from build123d import *

# Parameters (mm, degrees)
RESSALTO_EXTRUS_O1_DEPTH = 5


with BuildPart() as part:
    # Esboço1 → Ressalto-extrusão1 (new body)
    with BuildSketch(Plane.XY):
        with BuildLine():
            Line((0, 26.5), (0, 55.5))
            ThreePointArc((0, 55.5), (-9.054313021, 54.756455471), (-17.86602118, 52.545744711))
            Line((-17.86602118, 52.545744711), (-27.213841848, 24.565961853))
            Line((-27.213841848, 24.565961853), (-25.202997682, 8.188950351))
            Line((-25.202997682, 8.188950351), (-52.783636654, 17.150443188))
            ThreePointArc((-52.783636654, 17.150443188), (-54.874420381, 8.309511893), (-55.494877077, -0.754067766))
            Line((-55.494877077, -0.754067766), (-31.773157713, -18.290601927))
            Line((-31.773157713, -18.290601927), (-15.576309186, -21.438950351))
            Line((-15.576309186, -21.438950351), (-32.622081502, -44.900443188))
            ThreePointArc((-32.622081502, -44.900443188), (-24.859943887, -49.620894691), (-16.431699055, -53.01178422))
            Line((-16.431699055, -53.01178422), (7.576950452, -35.870175519))
            Line((7.576950452, -35.870175519), (15.576309186, -21.438950351))
            Line((15.576309186, -21.438950351), (32.622081502, -44.900443188))
            ThreePointArc((32.622081502, -44.900443188), (39.5101301, -38.976911364), (45.339528568, -32.009016686))
            Line((45.339528568, -32.009016686), (36.455970623, -3.878385726))
            Line((36.455970623, -3.878385726), (25.202997682, 8.188950351))
            Line((25.202997682, 8.188950351), (52.783636654, 17.150443188))
            ThreePointArc((52.783636654, 17.150443188), (49.278547189, 25.531838691), (44.453068744, 33.229123961))
            Line((44.453068744, 33.229123961), (14.954078486, 33.473201319))
            Line((14.954078486, 33.473201319), (0, 26.5))
        make_face()
        Polygon((-15.15, 8.746856578), (0, 17.493713156), (15.15, 8.746856578), (15.15, -8.746856578), (0, -17.493713156), (-15.15, -8.746856578), align=None, mode=Mode.SUBTRACT)
    extrude(amount=RESSALTO_EXTRUS_O1_DEPTH)


solid = part.part
Source: CAD feature listing. Evaluate the final solid. Frame: model axes, mm. A direction names the side the tool comes from. Round coordinates to 2 decimals unless told otherwise and drop trailing zeros. Loops run counter-clockwise (first coordinate to the right, second up) from the corner with the lowest first, then second, coordinate; pieces in that order, holes last. Notation, with made-up numbers: M 9.5,53 L 46.5,53 A26 cw 46.5,81 Z; hole C -10,73.25 d5. An arc over 180 degrees is marked long. Return JSON: item names as keys, results as strings. Group by question number.
1. Pin query (flat end, axial travel): pin 1 (1.5 mm diameter, centred on y = 45, z = 3.5, fed in from +X); pin 2 (2 mm diameter, centred on x = 2, z = 3.5, fed in from +Y); pin 3 (1.5 mm diameter, centred on y = -7, z = 2.5, fed in from -X); pin 4 (4 mm diameter, centred on x = -17.5, y = 8, fed in from -Z). Return the tip coordinate at first contact, or that it passes through.
2. Section query B-B on z = 4. Output: boundary loops of the cut face in (x, y), and give its area (3 significant figures).
3. Section query A-A on y = 3. Output: boundary loops of the cut face in (x, z).
4. Reachability of faces 4 (the face through (-23.788, -19.843, 2.465)), 5 (the face through (38.8, 12.607, 2.465)), 6 (the face through (-7.68, 13.06, 2.46)) from +Z, -Z, +X, -X, +Y, -Y: full face, straight path, thin tool, end or side. Return the list, or none.
5. Section query D-D on x = 17. Output: boundary loops of the cut face in (y, z), and give its area (3 significant figures).
6. Material intervals for line 1 along X through (y, z) = (-30, 0.3); line 2 along X through (y, z) = (-7.5, 0.8); line 3 along Y through (x, z) = (-30.5, 2.5), sorted ascending. Write a range as from..to.
7. Section query C-C on x = -20.5. Output: boundary loops of the cut face in (y, z).
8. Mould query, pull axis X, two halves, no side actions, for faces 1 (the face through (49.337, 25.419, 2.465)), 2 (the face through (-24.974, -49.564, 2.465)), 3 (the face through (11.52, -28.76, 2.46)). Classes: released by +X, released by -X, zero draft, split by the parting line, or undercut.
Checks:
{
 "1": {"pin 1": "stops at x = 0", "pin 2": "stops at y = 27.9", "pin 3": "stops at x = -48.06", "pin 4": "stops at z = 0"},
 "2": {"outline": "M -55.49,-0.75 L -31.77,-18.29 L -15.58,-21.44 L -32.62,-44.9 A55.5 ccw -16.43,-53.01 L 7.58,-35.87 L 15.58,-21.44 L 32.62,-44.9 A55.5 ccw 45.34,-32.01 L 36.46,-3.88 L 25.2,8.19 L 52.78,17.15 A55.5 ccw 44.45,33.23 L 14.95,33.47 L 0,26.5 L 0,55.5 A55.5 ccw -17.87,52.55 L -27.21,24.57 L -25.2,8.19 L -52.78,17.15 A55.5 ccw Z; hole M -15.15,-8.75 L 0,-17.49 L 15.15,-8.75 L 15.15,8.75 L 0,17.49 L -15.15,8.75 Z", "area": "5,200 mm²"},
 "3": {"outline": "M -55.42,0 L -15.15,0 L -15.15,5 L -55.42,5 Z; M 15.15,0 L 30.04,0 L 30.04,5 L 15.15,5 Z"},
 "4": {"face 4": "+Z, -Z, -X", "face 5": "+Z, -Z, +X", "face 6": "+Z, -Z"},
 "5": {"outline": "M -23.4,0 L 33.46,0 L 33.46,5 L -23.4,5 Z", "area": "284 mm²"},
 "6": {"line 1": "x = -21.8..10.83, 21.8..44.71", "line 2": "x = -46.37..-15.15, 15.15..37.6", "line 3": "y = -46.37..-41.98, -18.54..9.91"},
 "7": {"outline": "M -51.58,0 L -28.22,0 L -28.22,5 L -51.58,5 Z; M -20.48,0 L 44.66,0 L 44.66,5 L -20.48,5 Z"},
 "8": {"face 1": "released by +X", "face 2": "released by -X", "face 3": "undercut"}
}
